Autodesk Inventor part; units mm, degrees
ref_plane "YZ Plane" through (0, 0, 0) normal (1, 0, 0) x (0, 1, 0)
ref_plane "XZ Plane" through (0, 0, 0) normal (0, 1, 0) x (-1, 0, 0)
ref_plane "XY Plane" through (0, 0, 0) normal (0, 0, 1) x (1, 0, 0)
sketch "Sketch1" plane through (0, 0, 0) normal (0, 1, 0) x (-1, 0, 0)
  circle A0 centre (0, 0) radius 30
  circle A1 centre (0, 0) radius 22.5
  circle A2 centre (0, 0) radius 26.5
  circle A3 centre (0, 26.5) radius 2.15
  circle A4 centre (-26.5, 0) radius 2.15
  circle A5 centre (0, -26.5) radius 2.15
  circle A6 centre (26.5, 0) radius 2.15
  dimension "d3" = 53
  dimension "d0" = 60
  dimension "d1" = 45
  dimension "d4" = 4.3
  dimension "d7" = 360
extrude "Extrusion1" add sketch "Sketch1" against normal blind 4 contours A0 | A1 | A6 A2 A5 A4 A3
sketch "Sketch2" plane through (0, 0, 0) normal (0, 1, 0) x (1, 0, 0)
  circle A0 centre (0, 0) radius 20.5
  line L0 (-20.5, 0) -> (-20.5, 21.9032)
  circle A1 centre (0, 0) radius 30
  line L1 (20.5, 0) -> (20.5, 21.9032)
  circle A2 centre (0, 0) radius 30
  dimension "d11" = 41
extrude "Extrusion2" cut sketch "Sketch2" against normal blind 2.6 contours A0 | A0 L0 A1 L1 picked at (-0.8237, 26.6681)
sketch "Sketch3" plane through (0, -4, 0) normal (0, -1, 0) x (1, 0, 0)
  circle A0 centre (0, 0) radius 15
  dimension "d14" = 30
extrude "Extrusion3" cut sketch "Sketch3" against normal through all
sketch "Sketch4" plane through (0, -4, 0) normal (0, -1, 0) x (1, 0, 0)
  circle A0 centre (0, 0) radius 15
  circle A1 centre (0, 0) radius 17.5
  dimension "d17" = 30
  dimension "d18" = 35
extrude "Extrusion4" add sketch "Sketch4" along normal blind 8
properties part number "LoadCellMount"
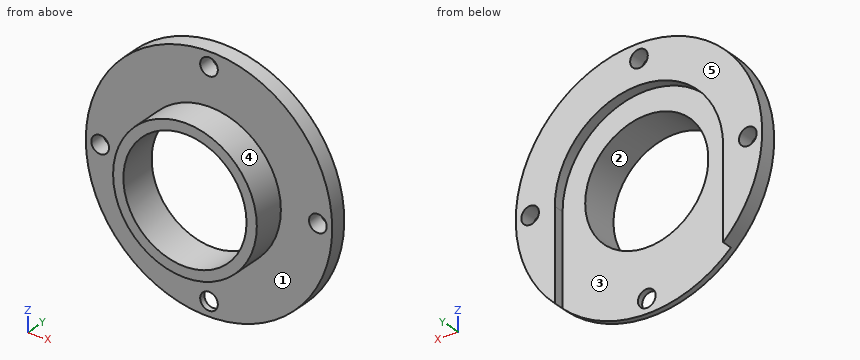
Model file for the job. Use its own axes, mm. Face numbers are marked on the shaded views. A direction names the side the tool comes from. Coordinates: 2 decimals unless noted, no trailing zeros. Order: outer loops, then holes, each group sorted by start corner. A loop starts at its lowest first (then second) coordinate and runs counter-clockwise, first axis right, second up. Notation, with made-up numbers: (-1, -15) -> (41, -15) arc R22 ccw to (41, -1) -> close; hole circle Ø1 at (-10, -38.75). An arc over 180 degrees is marked (long way). Return JSON: item names as keys, results as strings.
Item 1: Wall check: line 1 along Z through (x, y) = (0, -3.5); line 2 along X through (y, z) = (-1.9, 0); line 3 along Z through (x, y) = (0, -1.85). Give the ranges that are in metal, low to high. Write a range as from..to.
Model answer:
{"line 1": "z = -30..-28.65, -24.35..-15, 15..24.35, 28.65..30", "line 2": "x = -30..-28.65, -24.35..-20.5, 20.5..24.35, 28.65..30", "line 3": "z = 20.5..24.35, 28.65..30"}
Item 2: Slice it at C-C (z = -26.5). Write the cut outline in (x, y).
Model answer:
{"outline": "(-14.06, -4) -> (-2.15, -4) -> (-2.15, -2.6) -> (-14.06, -2.6) -> close; (2.15, -4) -> (14.06, -4) -> (14.06, -2.6) -> (2.15, -2.6) -> close"}
Item 3: 3-axis set-ups, long thin cutter, end or side, ignore diameter. For the marked faces 1 and 2: which of +Z, -Z, +X, -X, +Y, -Y reach the whole face in a straight line?
Model answer:
{"face 1": "-Y", "face 2": "+Y, -Y"}
Item 4: Slice it at B-B (y = -1). Write the cut outline in (x, z), then the cut area to 3 significant figures.
Model answer:
{"outline": "(-20.5, -21.9) -> (-20.5, 0) arc R20.5 cw to (20.5, 0) -> (20.5, -21.9) arc R30 ccw (long way) to start; hole circle Ø4.3 at (-26.5, 0); hole circle Ø4.3 at (0, 26.5); hole circle Ø4.3 at (26.5, 0)", "area": "998 mm²"}
Item 5: Slice it at D-D (x = -26.5). Write the cut outline in (y, z).
Model answer:
{"outline": "(-4, -14.06) -> (0, -14.06) -> (0, -2.15) -> (-4, -2.15) -> close; (-4, 2.15) -> (0, 2.15) -> (0, 14.06) -> (-4, 14.06) -> close"}
Item 6: Pin check, flat tips, straight feed: P1, Ø5, axis at x = 0, z = -26.5, coming from the +Y side; P2, Ø0.8, axis at y = -2, z = -10, coming from the -X side; P3, Ø3, axis at y = -1, z = -16, coming from the +X side. Stop position of each tip, or through.
Model answer:
{"P1": "stops at y = -2.6", "P2": "stops at x = -28.42", "P3": "stops at x = 26.26"}
Item 7: Mould opens along X. For the marked faces 3, 4 and 5 say: pulls with the +X half, pulls with the -X half, needs draft (parallel to the pull), parting line crosses it, or undercut.
Model answer:
{"face 3": "undercut", "face 4": "parting line crosses it", "face 5": "needs draft"}
Item 8: Slice it at A-A (x = 0). Write the cut outline in (y, z).
Model answer:
{"outline": "(-12, -17.5) -> (-4, -17.5) -> (-4, -24.35) -> (-2.6, -24.35) -> (-2.6, -15) -> (-12, -15) -> close; (-12, 15) -> (-2.6, 15) -> (-2.6, 20.5) -> (0, 20.5) -> (0, 24.35) -> (-4, 24.35) -> (-4, 17.5) -> (-12, 17.5) -> close; (-4, -30) -> (-2.6, -30) -> (-2.6, -28.65) -> (-4, -28.65) -> close; (-4, 28.65) -> (0, 28.65) -> (0, 30) -> (-4, 30) -> close"}
